from build123d import *

# Parameters (mm, degrees)
SKETCH1_R                      = 13
BOSS_EXTRUDE1_DEPTH            = 7
SKETCH2_R                      = 7.165
CUT_EXTRUDE1_DEPTH             = 5.15
SKETCH3_R                      = 3
BOSS_EXTRUDE2_DEPTH            = 12
FILLET1_R                      = 1
FILLET1_2_R                    = 0.5
CBORE_FOR_M3_SHCS1_D           = 3.6
CBORE_FOR_M3_SHCS1_DEPTH       = 7
CBORE_FOR_M3_SHCS1_CBORE_D     = 6.5
CBORE_FOR_M3_SHCS1_CBORE_DEPTH = 1.75
FILLET2_R                      = 0.5


with BuildPart() as part:
    # Sketch1 → Boss-Extrude1 (new body)
    with BuildSketch(Plane(origin=(0, 0, 0), x_dir=(1, 0, 0), z_dir=(0, 1, 0))):
        Circle(SKETCH1_R)
    extrude(amount=BOSS_EXTRUDE1_DEPTH)

    # Sketch2 → Cut-Extrude1 (cut)
    with BuildSketch(Plane.XZ):
        Circle(SKETCH2_R)
    extrude(amount=-CUT_EXTRUDE1_DEPTH, mode=Mode.SUBTRACT)

    # Sketch3 → Boss-Extrude2 (add)
    with BuildSketch(Plane(origin=(0, 7, 0), x_dir=(1, 0, 0), z_dir=(0, 1, 0))):
        Circle(SKETCH3_R)
    extrude(amount=BOSS_EXTRUDE2_DEPTH)

    # Fillet1
    fillet1_edges = [part.edges().sort_by_distance(p)[0] for p in [
        (-3, 7, 0),
    ]]
    fillet(fillet1_edges, radius=FILLET1_R)

    # Fillet1 2
    fillet1_2_edges = [part.edges().sort_by_distance(p)[0] for p in [
        (-13, 7, 0),
    ]]
    fillet(fillet1_2_edges, radius=FILLET1_2_R)

    # CBORE for M3 SHCS1
    with Locations(Plane(origin=(0, 7, 0), x_dir=(1, 0, 0), z_dir=(0, 1, 0))):
        with Locations((0, 9.5), (8.227241336, -4.75), (-8.227241336, -4.75)):
            CounterBoreHole(CBORE_FOR_M3_SHCS1_D / 2, CBORE_FOR_M3_SHCS1_CBORE_D / 2, CBORE_FOR_M3_SHCS1_CBORE_DEPTH, depth=CBORE_FOR_M3_SHCS1_DEPTH)

    # Fillet2
    fillet2_edges = [part.edges().sort_by_distance(p)[0] for p in [
        (-3, 19, 0),
        (-7.165, 0, 0),
    ]]
    fillet(fillet2_edges, radius=FILLET2_R)


solid = part.part
Work out the finished part from the listing and answer in its coordinate system (mm). A direction names the side the tool comes from. Give positions to 0.01 mm unless a question says otherwise; leave off trailing zeros. Write each loop counter-clockwise with the first axis right and the second up, starting at its lowest first coordinate (ties: lowest second). Pieces come first, ordered by that corner, then holes. Notation, with made-up numbers: M 69.25,60.25 L 125.25,60.25 A19 cw 125.25,68.25 Z; hole C 69.5,17.25 d3. An arc over 180 degrees is marked long. Answer as CSV lines item,"result".
Q1. A tool of negligible diameter and unlimited length cuts with its end or side. For faces 1 (the cylindrical face through (-3, 13, 0)), 2 (the cylindrical face through (-7.158, 2.792, 0.315)), 3 (the flat face through (0, 19, 0)), from which of +Z, -Z, +X, -X, +Y, -Y can it reach the whole face along a straight path? Write none if from no direction.
A:
face 1,"+Y"
face 2,"-Y"
face 3,"+Z, -Z, +X, -X, +Y"
Q2. A cutting plane is placed at A-A on z = 0. Write down the section's boundary in (x, y) (3 decimals).
A:
outline,"M -13,0 L -7.665,0 A0.5 ccw -7.165,0.5 L -7.165,5.15 L 7.165,5.15 L 7.165,0.5 A0.5 ccw 7.665,0 L 13,0 L 13,6.5 A0.5 ccw 12.5,7 L 4,7 A1 cw 3,8 L 3,18.5 A0.5 ccw 2.5,19 L -2.5,19 A0.5 ccw -3,18.5 L -3,8 A1 cw -4,7 L -12.5,7 A0.5 ccw -13,6.5 Z"
Q3. The mould has two halves that part along Z. Classify faces 4 (the flat face through (0, 5.15, 0)), 5 (the cylindrical face through (-10.316, 3.204, 7.91)), 6 (the flat face through (-3, 7, -3)): +Z half, -Z half, draft (parallel to the pull), parting line (faces both ways), or undercut.
A:
face 4,"undercut"
face 5,"parting line"
face 6,"draft"
Q4. A cutting plane is placed at C-C on x = 0. Write down the section's boundary in (y, z) (3 decimals).
A:
outline,"M 0,-13 L 6.5,-13 A0.5 ccw 6.933,-12.75 L 5.25,-12.75 L 5.25,-11.3 L 0,-11.3 Z; M 0,-7.7 L 5.25,-7.7 L 5.25,-6.25 L 7,-6.25 L 7,-4 A1 cw 8,-3 L 18.5,-3 A0.5 ccw 19,-2.5 L 19,2.5 A0.5 ccw 18.5,3 L 8,3 A1 cw 7,4 L 7,12.5 A0.5 ccw 6.5,13 L 0,13 L 0,7.665 A0.5 ccw 0.5,7.165 L 5.15,7.165 L 5.15,-7.165 L 0.5,-7.165 A0.5 ccw 0,-7.665 Z"
Q5. Given P1, Ø5, axis at x = 0.5, z = -2, coming from the -Y side; P2, Ø10.5, axis at x = -8.23, z = 4.75, coming from the +Y side; P3, Ø5, axis at x = 0.5, z = -9, coming from the +Y side, each flat-ended and moving along its own axis, determine where each tip first touches the part or whether it passes through.
A:
P1,"stops at y = 5.15"
P2,"stops at y = 7"
P3,"stops at y = 5.25"
Q6. Find the intervals of material crossed by probe 1 along Z at (x, y) = (0, 1.15) (3 decimals); probe 2 along Z at (x, y) = (-1, 1); probe 3 along Z at (x, y) = (0, 6.5), in increasing order. Write a range as [from, to].
A:
probe 1,"z = [-13, -11.3], [-7.7, -7.165], [7.165, 13]"
probe 2,"z = [-12.96, -11], [-8, -7.09], [7.09, 12.96]"
probe 3,"z = [-13, -12.75], [-6.25, 13]"
Q7. A cutting plane is placed at B-B on y = 1.5. Write down the section's boundary in (x, z) (3 decimals).
A:
outline,"C 0,0 d26; hole C -8.227,4.75 d3.6; hole C 0,0 d14.33; hole C 0,-9.5 d3.6; hole C 8.227,4.75 d3.6"
Q8. A cutting plane is placed at D-D on y = 9.25. Write down the section's boundary in (x, z).
A:
outline,"C 0,0 d6"
